```python
from build123d import *

# Parameters (mm, degrees)
SKETCH1_R           = 3.5
BOSS_EXTRUDE1_DEPTH = 7
CUT_EXTRUDE1_DEPTH  = 3
SKETCH3_W           = 13
SKETCH3_H           = 1.8
CUT_EXTRUDE2_DEPTH  = 4


with BuildPart() as part:
    # Sketch1 → Boss-Extrude1 (new body)
    with BuildSketch(Plane(origin=(0, 0, 0), x_dir=(0, 0, -1), z_dir=(1, 0, 0))):
        with BuildLine():
            Line((-12, 45), (-12, -45))
            ThreePointArc((-12, -45), (0, -57), (12, -45))
            Line((12, -45), (12, 45))
            ThreePointArc((12, 45), (0, 57), (-12, 45))
        make_face()
        with Locations((0, 45)):
            Circle(SKETCH1_R, mode=Mode.SUBTRACT)
        with Locations((0, -45)):
            Circle(SKETCH1_R, mode=Mode.SUBTRACT)
    extrude(amount=BOSS_EXTRUDE1_DEPTH)

    # Sketch2 → Cut-Extrude1 (cut)
    with BuildSketch(Plane(origin=(7, 0, 0), x_dir=(0, 0, -1), z_dir=(1, 0, 0))):
        with BuildLine():
            Line((-8.5, 45), (-8.5, 27))
            Line((-8.5, 27), (8.5, 27))
            Line((8.5, 27), (8.5, 45))
            ThreePointArc((8.5, 45), (0, 53.5), (-8.5, 45))
        make_face()
    extrude(amount=-CUT_EXTRUDE1_DEPTH, mode=Mode.SUBTRACT)

    # Sketch3 → Cut-Extrude2 (cut)
    with BuildSketch(Plane(origin=(7, 0, 0), x_dir=(0, 0, -1), z_dir=(1, 0, 0))):
        with Locations((0, -45)):
            Rectangle(SKETCH3_W, SKETCH3_H)
    extrude(amount=-CUT_EXTRUDE2_DEPTH, mode=Mode.SUBTRACT)


solid = part.part
```
Geometry check sheet. Reference: the model listing, model coordinates, mm. A direction names the side the tool comes from. Coordinates: 2 decimals unless noted, no trailing zeros. Order: outer loops, then holes, each group sorted by start corner. A loop starts at its lowest first (then second) coordinate and runs counter-clockwise, first axis right, second up. Notation, with made-up numbers: (-23, 66.25) - (-9, 66.25) arc R24 cw to (-9, 92.25) - close; hole circle Ø8 at (84, 58). An arc over 180 degrees is marked (long way). Answer in a Markdown table with one row per item. Add a question column.
1. Section check C-C (z = 10). Enter the section's corners in (x, y).
2. Material ranges on L1, parallel to Y at x = 2.45, z = 0; L2, parallel to Z at x = 1, y = 45; L3, parallel to Z at x = 3.5, y = -45, recorded low to high. Write a range as [from, to].
3. Section check B-B (y = 37). Enter the section's corners in (x, z).
4. Section check A-A (z = 0). Enter the section's corners in (x, y).
5. Gauge pin test, flat ends, axial feed: pin 1 Ø8.5 at (y, z) = (43.5, 0.5) entering from +X; pin 2 Ø3.5 at (x, z) = (4, -5) entering from +Y; pin 3 Ø1.6 at (x, z) = (5.5, 4.5) entering from -Y. Record the tip position at first contact, or that the pin passes through.
6. Draft check along Y on faces 1 (the face through (1.97, 48.47, 0.46)), 2 (the face through (3, 57, 0)), 3 (the face through (0, 1, 0)). Enter one of: +Y half, -Y half, draft (parallel to the pull), parting line (faces both ways), or undercut.
7. Access from +Z, -Z, +X, -X, +Y, -Y to the whole of each face (thin tool, end or side, straight path). Record for faces 4 (the face through (3.45, -43.95, -3.34)), 5 (the face through (5.521, 53.498, -0.187)).
Data:
| question | item | result |
|---|---|---|
| 1 | outline | (0, -51.63) - (7, -51.63) - (7, 51.63) - (0, 51.63) - close |
| 2 | L1 | y = [-57, -48.5], [-41.5, 41.5], [48.5, 57] |
| 2 | L2 | z = [-12, -3.5], [3.5, 12] |
| 2 | L3 | z = [-12, -6.5], [6.5, 12] |
| 3 | outline | (0, -12) - (7, -12) - (7, -8.5) - (4, -8.5) - (4, 8.5) - (7, 8.5) - (7, 12) - (0, 12) - close |
| 4 | outline | (0, -57) - (7, -57) - (7, -48.5) - (0, -48.5) - close; (0, -41.5) - (7, -41.5) - (7, 27) - (4, 27) - (4, 41.5) - (0, 41.5) - close; (0, 48.5) - (4, 48.5) - (4, 53.5) - (7, 53.5) - (7, 57) - (0, 57) - close |
| 5 | pin 1 | stops at x = 4 |
| 5 | pin 2 | stops at y = 56.55 |
| 5 | pin 3 | stops at y = -56.42 |
| 6 | face 1 | undercut |
| 6 | face 2 | +Y half |
| 6 | face 3 | draft |
| 7 | face 4 | +X, -X |
| 7 | face 5 | +X |
